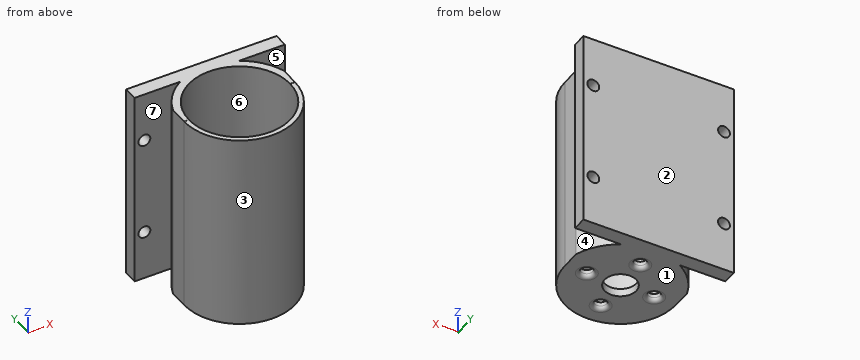
```python
from build123d import *

# Parameters (mm, degrees)
SKETCH1_R           = 14
BOSS_EXTRUDE1_DEPTH = 50
SKETCH5_W           = 28
SKETCH5_H           = 50.034880911
BOSS_EXTRUDE2_DEPTH = 21
SKETCH2_R           = 12.791811967
CUT_EXTRUDE1_DEPTH  = 48
SKETCH3_R           = 4
CUT_EXTRUDE2_DEPTH  = 49
SKETCH4_R           = 1.5
CUT_EXTRUDE3_DEPTH  = 49
SKETCH6_R           = 12.79
CUT_EXTRUDE5_DEPTH  = 21
SKETCH7_W           = 28
SKETCH7_H           = 4.634699127
CUT_EXTRUDE6_DEPTH  = 53
SKETCH8_W           = 50.034880911
SKETCH8_H           = 3.58
BOSS_EXTRUDE3_DEPTH = 5
SKETCH13_R          = 1.5
CUT_EXTRUDE7_DEPTH  = 5
SKETCH14_W          = 50.034880911
SKETCH14_H          = 3.58
BOSS_EXTRUDE4_DEPTH = 5
SKETCH15_R          = 1.5
CUT_EXTRUDE8_DEPTH  = 5
FILLET1_R           = 1
FILLET2_R           = 1
CUT_EXTRUDE9_DEPTH  = 73


with BuildPart() as part:
    # Sketch1 → Boss-Extrude1 (new body)
    with BuildSketch(Plane.XY):
        with Locations(Location((0, 0, 0), (0, 0, 180))):
            Circle(SKETCH1_R)
    extrude(amount=BOSS_EXTRUDE1_DEPTH)

    # Sketch5 → Boss-Extrude2 (add)
    with BuildSketch(Plane(origin=(0, 0, 0), x_dir=(1, 0, 0), z_dir=(0, 1, 0))):
        with Locations((0, -25.017440456)):
            Rectangle(SKETCH5_W, SKETCH5_H)
    extrude(amount=BOSS_EXTRUDE2_DEPTH)

    # Sketch2 → Cut-Extrude1 (cut)
    with BuildSketch(Plane.XY.offset(50)):
        Circle(SKETCH2_R)
    extrude(amount=-CUT_EXTRUDE1_DEPTH, mode=Mode.SUBTRACT)

    # Sketch3 → Cut-Extrude2 (cut)
    with BuildSketch(Plane(origin=(0, 0, 0), x_dir=(-1, 0, 0), z_dir=(0, 0, -1))):
        Circle(SKETCH3_R)
    extrude(amount=-CUT_EXTRUDE2_DEPTH, mode=Mode.SUBTRACT)

    # Sketch4 → Cut-Extrude3 (cut)
    with BuildSketch(Plane(origin=(0, 0, 0), x_dir=(-1, 0, 0), z_dir=(0, 0, -1))):
        with Locations((0, -8.5)):
            Circle(SKETCH4_R)
        with Locations((0, 8.5)):
            Circle(SKETCH4_R)
        with Locations((8.5, 0)):
            Circle(SKETCH4_R)
        with Locations((-8.5, 0)):
            Circle(SKETCH4_R)
    extrude(amount=-CUT_EXTRUDE3_DEPTH, mode=Mode.SUBTRACT)

    # Sketch6 → Cut-Extrude5 (cut)
    with BuildSketch(Plane.XY.offset(50.034880911)):
        Circle(SKETCH6_R)
    extrude(amount=-CUT_EXTRUDE5_DEPTH, mode=Mode.SUBTRACT)

    # Sketch7 → Cut-Extrude6 (cut)
    with BuildSketch(Plane.XY.offset(50.034880911)):
        with Locations((0, 18.682650437)):
            Rectangle(SKETCH7_W, SKETCH7_H)
    extrude(amount=-CUT_EXTRUDE6_DEPTH, mode=Mode.SUBTRACT)

    # Sketch8 → Boss-Extrude3 (add)
    with BuildSketch(Plane(origin=(14, 0, 0), x_dir=(0, 0, -1), z_dir=(1, 0, 0))):
        with Locations((-25.017440456, 14.575300873)):
            Rectangle(SKETCH8_W, SKETCH8_H)
    extrude(amount=BOSS_EXTRUDE3_DEPTH)

    # Sketch13 → Cut-Extrude7 (cut)
    with BuildSketch(Plane.XZ.offset(-12.785300873)):
        with Locations(Location((16.5, 37.526160683, 0), (0, 0, 270))):
            Circle(SKETCH13_R)
        with Locations(Location((16.5, 12.508720228, 0), (0, 0, 270))):
            Circle(SKETCH13_R)
    extrude(amount=-CUT_EXTRUDE7_DEPTH, mode=Mode.SUBTRACT)

    # Sketch14 → Boss-Extrude4 (add)
    with BuildSketch(Plane.ZY.offset(14)):
        with Locations((25.017440456, 14.575300873)):
            Rectangle(SKETCH14_W, SKETCH14_H)
    extrude(amount=BOSS_EXTRUDE4_DEPTH)

    # Sketch15 → Cut-Extrude8 (cut)
    with BuildSketch(Plane.XZ.offset(-12.785300873)):
        with Locations(Location((-16.5, 12.508720228, 0), (0, 0, 270))):
            Circle(SKETCH15_R)
        with Locations(Location((-16.5, 37.526160683, 0), (0, 0, 270))):
            Circle(SKETCH15_R)
    extrude(amount=-CUT_EXTRUDE8_DEPTH, mode=Mode.SUBTRACT)

    # Fillet1
    fillet1_edges = [part.edges().sort_by_distance(p)[0] for p in [
        (10, 0, 0),
    ]]
    fillet(fillet1_edges, radius=FILLET1_R)

    # Fillet2
    fillet2_edges = [part.edges().sort_by_distance(p)[0] for p in [
        (1.5, -8.5, 0),
        (1.5, 8.5, 0),
        (-7, 0, 0),
    ]]
    fillet(fillet2_edges, radius=FILLET2_R)

    # Sketch16 → Cut-Extrude9 (cut)
    with BuildSketch(Plane(origin=(0, 0, 0), x_dir=(-1, 0, 0), z_dir=(0, 0, -1))):
        with BuildLine():
            Line((-7.445480913, 12.785300873), (-14, 12.785300873))
            Line((-14, 12.785300873), (-14, 4.785300873))
            ThreePointArc((-14, 4.785300873), (-11.444525455, 9.376670067), (-7.445480913, 12.785300873))
        make_face()
        with BuildLine():
            Line((14, 12.785300873), (14, 4.785300873))
            ThreePointArc((14, 4.785300873), (11.444525455, 9.376670067), (7.445480913, 12.785300873))
            Line((7.445480913, 12.785300873), (14, 12.785300873))
        make_face()
    extrude(amount=-CUT_EXTRUDE9_DEPTH, mode=Mode.SUBTRACT)


solid = part.part
```
Build history of the part. All positions in model axes, mm. Face numbers are marked on the shaded views. A direction names the side the tool comes from. Give positions to 0.01 mm unless a question says otherwise; leave off trailing zeros. Loops run counter-clockwise (first coordinate to the right, second up) from the corner with the lowest first, then second, coordinate; pieces in that order, holes last. Notation, with made-up numbers: (50.5, 69.5) - (58.5, 69.5) arc R20 ccw to (58.5, 83.5) - close; hole circle Ø6 at (-38.5, 65.5). An arc over 180 degrees is marked (long way). Use a Markdown table: item, result.
(1) Which spindle directions (+Z, -Z, +X, -X, +Y, -Y) get a long thin tool onto all of the face, cutting with end or side? Do the marked faces 5, 6 and 7. Say none if no direction does.
Taken from the geometry:
| item | result |
|---|---|
| face 5 | +Z, -Z, +X |
| face 6 | +Z |
| face 7 | +Z, -Z, -X |
(2) Band-saw the part on A-A (z = 28). Give the cut face in (x, y).
Taken from the geometry:
| item | result |
|---|---|
| outline | (-19, 12.79) - (-7.45, 12.79) arc R14.8 ccw to (-14, 4.79) - (-14, 0) arc R14 ccw to (14, 0) - (14, 4.79) arc R14.8 ccw to (7.45, 12.79) - (19, 12.79) - (19, 16.37) - (-19, 16.37) - close; hole circle Ø25.58 at (0, 0) |
(3) Wall check: line 1 along Y through (x, z) = (11, 19); line 2 along Y through (x, z) = (-8.5, 1.6); line 3 along X through (y, z) = (0.5, 23). Give the ranges that are in metal, low to high.
Taken from the geometry:
| item | result |
|---|---|
| line 1 | -8.66 to -6.53, 6.53 to 9.89, 12.79 to 16.37 |
| line 2 | -11.12 to -1.5, 1.5 to 12.11, 12.79 to 16.37 |
| line 3 | -14 to -12.78, 12.78 to 14 |
(4) Drop flat-ended pins along their axis: pin 1 Ø3.5 at (x, z) = (16.5, 37.53) entering from -Y; pin 2 Ø1 at (x, y) = (8, -7) entering from +Z; pin 3 Ø6 at (x, z) = (-14, 24.5) entering from -Y; pin 4 Ø2.5 at (x, z) = (-16.5, 12.51) entering from +Y. Give the stop position or say it passes through.
Taken from the geometry:
| item | result |
|---|---|
| pin 1 | y = 12.79 |
| pin 2 | z = 2 |
| pin 3 | y = -8.66 |
| pin 4 | through |
(5) Band-saw the part on B-B (x = -16.5). Give the cut face in (y, z), and give its area (3 significant figures).
Taken from the geometry:
| item | result |
|---|---|
| outline | (12.79, 0) - (16.37, 0) - (16.37, 11.01) - (12.79, 11.01) - close; (12.79, 14.01) - (16.37, 14.01) - (16.37, 36.03) - (12.79, 36.03) - close; (12.79, 39.03) - (16.37, 39.03) - (16.37, 50.03) - (12.79, 50.03) - close |
| area | 158 mm2 |
(6) Band-saw the part on C-C (z = 12). Give the cut face in (x, y), and give its area (3 significant figures).
Taken from the geometry:
| item | result |
|---|---|
| outline | (-19, 12.79) - (-17.91, 12.79) - (-17.91, 16.37) - (-19, 16.37) - close; (-15.09, 12.79) - (-7.45, 12.79) arc R14.8 ccw to (-14, 4.79) - (-14, 0) arc R14 ccw to (14, 0) - (14, 4.79) arc R14.8 ccw to (7.45, 12.79) - (15.09, 12.79) - (15.09, 16.37) - (-15.09, 16.37) - close; (17.91, 12.79) - (19, 12.79) - (19, 16.37) - (17.91, 16.37) - close; hole circle Ø25.58 at (0, 0) |
| area | 228 mm2 |
(7) Pull direction Y, two halves, no side cores. Call the marked faces 1, 2, 3 and 4: +Y half, -Y half, draft (parallel to the pull), parting line (faces both ways), or undercut.
Taken from the geometry:
| item | result |
|---|---|
| face 1 | draft |
| face 2 | +Y half |
| face 3 | -Y half |
| face 4 | undercut |
